The listing builds one solid part. Answer for the finished solid, in the listing's coordinates (mm). A direction names the side the tool comes from. Coordinates: 2 decimals unless noted, no trailing zeros. Order: outer loops, then holes, each group sorted by start corner. A loop starts at its lowest first (then second) coordinate and runs counter-clockwise, first axis right, second up. Notation, with made-up numbers: (69, 7.25) -> (85, 7.25) arc R18 cw to (85, 13.25) -> close; hole circle Ø4 at (74, 80.5). An arc over 180 degrees is marked (long way). Write item = value, one per line.
from build123d import *

# Parameters (mm, degrees)
F1_DEPTH       = 20
F2_R           = 30
F3_DEPTH       = 50
F4_R           = 25
F5_DEPTH       = 40
F7_D           = 8.8
F7_CBORE_D     = 14.25
F7_CBORE_DEPTH = 8
F8_R           = 5
F9_DEPTH       = 30.001
F10_R          = 7.5
F11_DEPTH      = 10
F12_R          = 15


# Not quite as in the source:
# - a pattern or mirror of a feature is missing from the dataset's text; its kind, count and spacing are read off the source's solid


with BuildPart() as f1:
    # F0 (on Top) → F1 (new body)
    with BuildSketch(Plane.XY):
        with BuildLine():
            Line((-45, -20), (45, -20))
            ThreePointArc((45, -20), (65, 0), (45, 20))
            Line((45, 20), (-45, 20))
            ThreePointArc((-45, 20), (-65, 0), (-45, -20))
        make_face()
    extrude(amount=F1_DEPTH)

    # F2 (on Top) → F3 (join)
    with BuildSketch(Plane.XY):
        Circle(F2_R)
    extrude(amount=F3_DEPTH)

    # F4 (on face) → F5 (cut)
    with BuildSketch(Plane.XY.offset(50)):
        Circle(F4_R)
    extrude(amount=-F5_DEPTH, mode=Mode.SUBTRACT)

    # F7 (through all)
    with Locations(Plane.XY.offset(20)):
        with Locations((45, 0)):
            f7 = CounterBoreHole(F7_D / 2, F7_CBORE_D / 2, F7_CBORE_DEPTH)

    # F7_copies: F7 across plane
    add(f7.mirror(Plane(origin=(0, 0, 0), x_dir=(0, 0, -1), z_dir=(-1, 0, 0))), mode=Mode.SUBTRACT)

    # F8 (on Front) → F9 (cut, through all)
    with BuildSketch(Plane.XZ):
        with Locations((0, 30)):
            Circle(F8_R)
    extrude(amount=F9_DEPTH, mode=Mode.SUBTRACT)

    # F10 (on face) → F11 (cut, through all)
    with BuildSketch(Plane.XY.offset(10)):
        Circle(F10_R)
    extrude(amount=-F11_DEPTH, mode=Mode.SUBTRACT)

    # F12
    f12_edges = [f1.edges().sort_by_distance(p)[0] for p in [
        (-22.36068, -20, 10),
        (22.36068, -20, 10),
        (-22.36068, 20, 10),
        (22.36068, 20, 10),
    ]]
    fillet(f12_edges, radius=F12_R)


solid = f1.part
Q1. Section C-C, the plane x = 43 is taken. Give the vertices of the cut face in (y, z).
The answers:
outline = (-20, 0) -> (-3.92, 0) -> (-3.92, 12) -> (-6.84, 12) -> (-6.84, 20) -> (-20, 20) -> close; (3.92, 0) -> (20, 0) -> (20, 20) -> (6.84, 20) -> (6.84, 12) -> (3.92, 12) -> close
Q2. Find the intervals of material crossed by line 1 along Y through (x, z) = (-45, 13.5) (3 decimals); line 2 along Y through (x, z) = (0, 7); line 3 along Z through (x, y) = (16.5, -11), in increasing order.
The answers:
line_1 = -20 to -7.125, 7.125 to 20
line_2 = -30 to -7.5, 7.5 to 30
line_3 = 0 to 10
Q3. A tool of negligible diameter and unlimited length cuts with its end or side. For faces 5 (the face through (-5, -27, 30)), 6 (the face through (-51.796, 2.14, 16.056)), 7 (the face through (-1, -13, 0)), 8 (the face through (-37, 20, 10)), from which of +Z, -Z, +X, -X, +Y, -Y can it reach the whole face along a straight path? Write none if from no direction.
The answers:
face_5 = -Y
face_6 = +Z
face_7 = -Z, +X, -X, +Y, -Y
face_8 = +Z, -Z, -X, +Y
Q4. The mould has two halves that part along Y. Classify faces 1 (the face through (36, 0, 20)), 2 (the face through (23.22, 20.88, 9.86)), 3 (the face through (28.615, 9.011, 30.206)), 4 (the face through (23.846, 7.509, 30.28)): released by +Y, released by -Y, zero draft, split by the parting line, or undercut.
The answers:
face_1 = zero draft
face_2 = released by +Y
face_3 = split by the parting line
face_4 = undercut
Q5. Section D-D, the plane z = 14.5 is taken. Give the vertices of the cut face in (x, y) (3 decimals).
The answers:
outline = (-45, -20) -> (-28.284, -20) arc R15 cw to (-18.856, -23.333) arc R30 ccw to (18.856, -23.333) arc R15 cw to (28.284, -20) -> (45, -20) arc R20 ccw to (45, 20) -> (28.284, 20) arc R15 cw to (18.856, 23.333) arc R30 ccw to (-18.856, 23.333) arc R15 cw to (-28.284, 20) -> (-45, 20) arc R20 ccw to start; hole circle Ø14.25 at (-45, 0); hole circle Ø50 at (0, 0); hole circle Ø14.25 at (45, 0)
Q6. Section A-A, the plane z = 5 is taken. Give the vertices of the cut face in (x, y).
The answers:
outline = (-45, -20) -> (-28.28, -20) arc R15 cw to (-18.86, -23.33) arc R30 ccw to (18.86, -23.33) arc R15 cw to (28.28, -20) -> (45, -20) arc R20 ccw to (45, 20) -> (28.28, 20) arc R15 cw to (18.86, 23.33) arc R30 ccw to (-18.86, 23.33) arc R15 cw to (-28.28, 20) -> (-45, 20) arc R20 ccw to start; hole circle Ø8.8 at (-45, 0); hole circle Ø15 at (0, 0); hole circle Ø8.8 at (45, 0)
Q7. Section B-B, the plane y = 0 is taken. Give the number of separate pieces and of enclosed holes in the cut face, plus the area to 3 significant figures.
The answers:
separate_pieces = 4
enclosed_holes = 0
area = 1,810 mm2
Q8. Each of these flat-tipped pins is pushed along its axis until it touches: pin 1 Ø25 at (x, y) = (5.5, 3) entering from +Z; pin 2 Ø8 at (y, z) = (-15.5, 26) entering from +X; pin 3 Ø13.5 at (x, z) = (36, 12.5) entering from -Y. Where does it stop, or does it pass through?
The answers:
pin_1 = 10
pin_2 = 27.71
pin_3 = -20
